```python
from build123d import *

# Parameters (mm, degrees)
CYLINDER005_R     = 1.6
CYLINDER005_DEPTH = 30
PAD001_DEPTH      = 13
SKETCH001_W       = 28
SKETCH001_H       = 4.4
POCKET002_DEPTH   = 7.4


with BuildPart() as finger_drill_master:
    # Cylinder005 → Cylinder005 (new body)
    with BuildSketch(Plane.XY.offset(-8)):
        Circle(CYLINDER005_R)
    extrude(amount=CYLINDER005_DEPTH)


with BuildPart() as clone001:
    # Clone001 base: copy of finger-drill-master
    add(finger_drill_master.part)


with BuildPart() as clone001_1:
    # Clone001 placement: moved
    add(clone001.part.moved(Location((-5.5, 28.9, 0))))


with BuildPart() as finger_drills:
    # Clone002 base: copy of finger-drill-master
    add(finger_drill_master.part)


with BuildPart() as finger_drills_1:
    # Clone002 placement: moved
    add(finger_drills.part.moved(Location((-13.5, 44.9, 0))))

    # Fusion011: union Clone001
    add(clone001_1.part)


with BuildPart() as clone_of_left_finger:
    # Sketch007 → Pad001 (new body)
    with BuildSketch(Plane.XY):
        with BuildLine():
            Line((0, 0), (0, 18))
            Line((0, 18), (-5.5, 18))
            Line((-5.5, 18), (-5.5, 25.2))
            ThreePointArc((-5.5, 25.2), (-2.3525883805, 26.9548007564), (-2.1906255667, 30.55470265))
            Line((-10.1906192745, 46.5546900658), (-2.1906255667, 30.55470265))
            ThreePointArc((-10.1906192745, 46.5546900658), (-14.7496924515, 48.3825664066), (-17.1063967324, 44.0730159565))
            Line((-17.1063967324, 44.0730159565), (-7, 0))
            Line((-7, 0), (0, 0))
        make_face()
    extrude(amount=PAD001_DEPTH)

    # Sketch001 → Pocket002 (cut)
    with BuildSketch(Plane(origin=(10.4693806066, 5.2346903033, 0), x_dir=(-0.4472135955, 0.894427191, 0), z_dir=(0.894427191, 0.4472135955, 0))):
        with Locations((37.2528992744, 6.5)):
            Rectangle(SKETCH001_W, SKETCH001_H)
    extrude(amount=-POCKET002_DEPTH, mode=Mode.SUBTRACT)

    # Cut012: cut finger-drills
    add(finger_drills_1.part, mode=Mode.SUBTRACT)


with BuildPart() as clone_of_left_finger_1:
    # Cut012 placement: moved
    add(clone_of_left_finger.part.moved(Location((0, -57, 0))))


with BuildPart() as clone_of_left_finger_2:
    # Clone003 placement: moved
    add(clone_of_left_finger_1.part.moved(Location((192.6034801236, 242.5662976869, 0))))


with BuildPart() as clone_of_left_finger_3:
    # Clone180 placement: moved
    add(clone_of_left_finger_2.part.moved(Location((-14.0004801236, -699.0002976869, 18.3))))


solid = clone_of_left_finger_3.part
```
Work out the finished part from the listing and answer in its coordinate system (mm). A direction names the side the tool comes from. Round coordinates to 2 decimals unless told otherwise and drop trailing zeros. Write each loop counter-clockwise with the first axis right and the second up, starting at its lowest first coordinate (ties: lowest second). Pieces come first, ordered by that corner, then holes.
1) Determine the mould class of faces 1 (the face through (170, -489, 18.3)), 2 (the face through (176.222, -486.524, 29.12)), 3 (the face through (172.586, -490.445, 24.769)) for opening direction Z: pulls with the +Z half, pulls with the -Z half, needs draft (parallel to the pull), parting line crosses it, or undercut.
2) A cutting plane is placed at A-A on z = 23.25. Determine the outline of the cut face in (x, y), and give its area (3 significant figures).
3) A cutting plane is placed at D-D on x = 169.5. Determine the outline of the cut face in (y, z).
4) Which of the six approach directions +Z, -Z, +X, -X, +Y, -Y give full straight-line access (tool end or side, diameter ignored) to faces 4 (the face through (173.103, -492, 25)), 5 (the face through (172.756, -486.096, 20.42))?
5) Consider probe 1 along Z at (x, y) = (162.5, -469); probe 2 along Y at (x, z) = (172.75, 30.5); probe 3 along X at (y, z) = (-500, 24.5). Determine where each line is inside the solid, lowest interval first.
6) A cutting plane is placed at B-B on z = 30. Determine the outline of the cut face in (x, y).
7) A cutting plane is placed at C-C on x = 175.25. Determine the outline of the cut face in (y, z).
8) A flat-ended cylindrical pin translates along its axis: P1, Ø5, axis at x = 171, z = 26.5, coming from the +Y side. Find the tip coordinate at first contact, or state that the pin passes through.
Entries:
1. face 1: pulls with the -Z half
1. face 2: needs draft
1. face 3: undercut
2. outline: (161.6, -469.79) - (171.6, -513.43) - (178.6, -513.43) - (178.6, -495.43) - (173.1, -495.43) - (173.1, -490.19) - (172.05, -490.71) - close
2. area: 252 mm2
3. outline: (-504.26, 18.3) - (-469.05, 18.3) - (-469.05, 22.6) - (-485.6, 22.6) - (-485.6, 27) - (-469.05, 27) - (-469.05, 31.3) - (-504.26, 31.3) - close
4. face 4: +Z, -Z, +X
4. face 5: +Z, -Z
5. probe 1: z = 18.3 to 22.6, 27 to 31.3
5. probe 2: y = -513.43 to -486.09, -482.97 to -475.55
5. probe 3: x = 168.52 to 178.6
6. outline: (161.5, -469.36) - (171.6, -513.43) - (178.6, -513.43) - (178.6, -495.43) - (173.1, -495.43) - (173.1, -488.23) arc R3.7 ccw to (176.41, -482.88) - (168.41, -466.88) arc R3.7 ccw to start; hole circle Ø3.2 at (165.1, -468.53); hole circle Ø3.2 at (173.1, -484.53)
7. outline: (-513.43, 18.3) - (-495.43, 18.3) - (-495.43, 31.3) - (-513.43, 31.3) - close; (-487.55, 18.3) - (-480.55, 18.3) - (-480.55, 22.6) - (-487.55, 22.6) - close; (-487.55, 27) - (-480.55, 27) - (-480.55, 31.3) - (-487.55, 31.3) - close
8. P1: stops at y = -467.16
